Here's how the part is built. I have some questions about the finished solid (model axes, mm). A direction names the side the tool comes from. Coordinates: 2 decimals unless noted, no trailing zeros. Write each loop counter-clockwise with the first axis right and the second up, starting at its lowest first coordinate (ties: lowest second). Pieces come first, ordered by that corner, then holes.
Item 1: For faces 1 (the face through (9, -12, -5)), 2 (the face through (9, -12, -4)), which set-ups out of +Z, -Z, +X, -X, +Y, -Y let a thin tool reach every point of the face, with its end or its side?
Item 2: If we section it at B-B (y = -12.5): Please give me the cut outline in (x, z).
Item 3: If we section it at C-C (x = 9): Please give me the cut outline in (y, z), then the cut area to 3 significant figures.
Item 4: If I drill on line 1 (Y direction, x = 9, z = -1.5); line 2 (Z direction, x = 13.5, y = -20.75); line 3 (X direction, y = -9, z = -2.15), over which ranges is the centre line in solid material (lowest first)?
Item 5: We'd pull the mould along X, two halves only. Please class faces 3 (the face through (9.508, -13.476, -2.028)), 4 (the face through (18.061, -9.646, -2.518)), 5 (the face through (9, -14, 0)): +X half, -X half, draft (parallel to the pull), parting line (faces both ways), or undercut.
Item 6: I'm going to push flat-ended pins straight in: pin 1 Ø1 at (x, z) = (9, -0.5) entering from +Y; pin 2 Ø1 at (x, z) = (7.5, -4) entering from +Y. Where does each tip first touch, or does it pass through?
Item 7: If we section it at A-A (z = -2.75): Please give me the cut outline in (x, y).
Item 8: If we section it at D-D (z = -4.55): Please give me the cut outline in (x, y).
from build123d import *

# Parameters (mm, degrees)
CYLINDER013_R     = 1.1
CYLINDER013_DEPTH = 5
CYLINDER012_R     = 9.5
CYLINDER012_DEPTH = 5
FILLET002003_R    = 1.2


with BuildPart() as footbase001:
    # Cylinder013 → Cylinder013 (new body)
    with BuildSketch(Plane(origin=(9, 9.5, -4), x_dir=(1, 0, 0), z_dir=(0, 0, 1))):
        Circle(CYLINDER013_R)
    extrude(amount=CYLINDER013_DEPTH)


with BuildPart() as foot:
    # Cylinder012 → Cylinder012 (new body)
    with BuildSketch(Plane(origin=(9, 9.5, -5), x_dir=(1, 0, 0), z_dir=(0, 0, 1))):
        Circle(CYLINDER012_R)
    extrude(amount=CYLINDER012_DEPTH)

    # Cut001002: cut FootBase001
    add(footbase001.part, mode=Mode.SUBTRACT)


with BuildPart() as foot_1:
    # Cut001002 placement: moved
    add(foot.part.moved(Location((0, -22, 0))))

    # Fillet002003
    fillet002003_edges = [foot_1.edges().sort_by_distance(p)[0] for p in [
        (-0.5, -12.5, 0),
        (-0.5, -12.5, -5),
    ]]
    fillet(fillet002003_edges, radius=FILLET002003_R)


solid = foot_1.part
Answer list:
1. face 1: -Z, +X, -X, +Y, -Y
1. face 2: +Z
2. outline: (-0.5, -3.8) arc R1.2 ccw to (0.7, -5) - (17.3, -5) arc R1.2 ccw to (18.5, -3.8) - (18.5, -1.2) arc R1.2 ccw to (17.3, 0) - (10.1, 0) - (10.1, -4) - (7.9, -4) - (7.9, 0) - (0.7, 0) arc R1.2 ccw to (-0.5, -1.2) - close
3. outline: (-22, -3.8) arc R1.2 ccw to (-20.8, -5) - (-4.2, -5) arc R1.2 ccw to (-3, -3.8) - (-3, -1.2) arc R1.2 ccw to (-4.2, 0) - (-11.4, 0) - (-11.4, -4) - (-13.6, -4) - (-13.6, 0) - (-20.8, 0) arc R1.2 ccw to (-22, -1.2) - close
3. area: 85.0 mm2
4. line 1: y = -22 to -13.6, -11.4 to -3
4. line 2: z = -4.29 to -0.71
4. line 3: x = 0.17 to 17.83
5. face 3: undercut
5. face 4: parting line
5. face 5: draft
6. pin 1: stops at y = -3.02
6. pin 2: stops at y = -3.06
7. outline: circle Ø19 at (9, -12.5); hole circle Ø2.2 at (9, -12.5)
8. outline: circle Ø18.47 at (9, -12.5)
